```python
from build123d import *

# Parameters (mm, degrees)
ESQUISSE1_R             = 35
ESQUISSE1_R_2           = 7
BOSS_EXTRU_1_DEPTH      = 20
ESQUISSE2_R             = 14
ENL_V_MAT_EXTRU_1_DEPTH = 5
ESQUISSE3_R             = 4
ENL_V_MAT_EXTRU_3_DEPTH = 5
ESQUISSE8_R             = 14
ENL_V_MAT_EXTRU_4_DEPTH = 25
BOSS_EXTRU_2_DEPTH      = 6
BOSS_EXTRU_2_DEPTH_BACK = 9
ESQUISSE9_R             = 4
ESQUISSE10_R            = 14
ESQUISSE10_R_2          = 10.5
BOSS_EXTRU_3_DEPTH      = 20


with BuildPart() as part:
    # Esquisse1 → Boss.-Extru.1 (new body)
    with BuildSketch(Plane.XY):
        Circle(ESQUISSE1_R)
        Circle(ESQUISSE1_R_2, mode=Mode.SUBTRACT)
    extrude(amount=BOSS_EXTRU_1_DEPTH)

    # Esquisse2 → Enlèv. mat.-Extru.1 (cut)
    with BuildSketch(Plane(origin=(0, 0, 0), x_dir=(-1, 0, 0), z_dir=(0, 0, -1))):
        Circle(ESQUISSE2_R)
    extrude(amount=-ENL_V_MAT_EXTRU_1_DEPTH, mode=Mode.SUBTRACT)

    # Esquisse3 → Enlèv. mat.-Extru.3 (cut)
    with BuildSketch(Plane(origin=(0, 0, 0), x_dir=(-1, 0, 0), z_dir=(0, 0, -1))):
        with Locations((-13.588993608, 22.602101614)):
            Circle(ESQUISSE3_R)
        with Locations((13.588993608, 22.602101614)):
            Circle(ESQUISSE3_R)
        with Locations((26.369096609, 0.431843358)):
            Circle(ESQUISSE3_R)
        with Locations((12.841601354, -23.034952123)):
            Circle(ESQUISSE3_R)
        with Locations((-12.82933858, -23.041784138)):
            Circle(ESQUISSE3_R)
        with Locations((-26.369096609, 0.431843358)):
            Circle(ESQUISSE3_R)
    extrude(amount=-ENL_V_MAT_EXTRU_3_DEPTH, mode=Mode.SUBTRACT)

    # Esquisse8 → Enlèv. mat.-Extru.4 (cut)
    with BuildSketch(Plane(origin=(0, 0, 0), x_dir=(-1, 0, 0), z_dir=(0, 0, -1))):
        Circle(ESQUISSE8_R)
    extrude(amount=-ENL_V_MAT_EXTRU_4_DEPTH, mode=Mode.SUBTRACT)

    # Esquisse9 → Boss.-Extru.2 (add, two sides: drawn at the far end of the back side and taken through both)
    with BuildSketch(Plane(origin=(0, 0, 0), x_dir=(-1, 0, 0), z_dir=(0, 0, -1)).offset(-BOSS_EXTRU_2_DEPTH_BACK)):
        with Locations((-13.588993608, 22.602101614)):
            Circle(ESQUISSE9_R)
        with Locations((13.588993608, 22.602101614)):
            Circle(ESQUISSE9_R)
        with Locations((26.369096609, 0.431843358)):
            Circle(ESQUISSE9_R)
        with Locations((12.841601354, -23.034952123)):
            Circle(ESQUISSE9_R)
        with Locations((-12.82933858, -23.041784138)):
            Circle(ESQUISSE9_R)
        with Locations((-26.369096609, 0.431843358)):
            Circle(ESQUISSE9_R)
    extrude(amount=BOSS_EXTRU_2_DEPTH + BOSS_EXTRU_2_DEPTH_BACK)

    # Esquisse10 → Boss.-Extru.3 (add)
    with BuildSketch(Plane(origin=(0, 0, 0), x_dir=(-1, 0, 0), z_dir=(0, 0, -1))):
        Circle(ESQUISSE10_R)
        Circle(ESQUISSE10_R_2, mode=Mode.SUBTRACT)
    extrude(amount=-BOSS_EXTRU_3_DEPTH)


solid = part.part
```
Model file for the job. Use its own axes, mm. A direction names the side the tool comes from. Give positions to 0.01 mm unless a question says otherwise; leave off trailing zeros. Order: outer loops, then holes, each group sorted by start corner. A loop starts at its lowest first (then second) coordinate and runs counter-clockwise, first axis right, second up.
1) Saw through at D-D, the plane x = 14.5. Write the cut outline in (y, z), then the cut area to 3 significant figures.
2) Saw through at B-B, the plane z = -1.75. Write the cut outline in (x, y), then the cut area to 3 significant figures.
3) Mould opens along X. For faces 3 (the cylindrical face through (22.674, -1.1, -2.958)), 4 (the cylindrical face through (9.014, -21.84, -2.958)), 5 (the flat face through (14, 23, -6)), 6 (the cylindrical face through (-28, -21, 10)) say: +X half, -X half, draft (parallel to the pull), parting line (faces both ways), or undercut.
4) Saw through at C-C, the plane y = -2. Write the cut outline in (x, z).
5) Pin check, flat tips, straight feed: pin 1 (6 mm diameter, centred on x = -4.5, z = 9.5, fed in from -Y); pin 2 (1.5 mm diameter, centred on y = 21, z = 14, fed in from -X); pin 3 (2 mm diameter, centred on x = -4.5, z = 0, fed in from -Y); pin 4 (17 mm diameter, centred on x = 0, y = 0, fed in from -Z). Stop position of each tip, or through.
6) Wall check: probe 1 along Y at (x, z) = (0, 5); probe 2 along Z at (x, y) = (7, 22.5); probe 3 along Y at (x, z) = (5.5, 6.75). Give the ranges that are in metal, low to high.
7) 3-axis set-ups, long thin cutter, end or side, ignore diameter. For faces 1 (the flat face through (-26, 0, -6)), 2 (the flat face through (8.3, -7.3, 0)): which of +Z, -Z, +X, -X, +Y, -Y reach the whole face in a straight line?
8) Saw through at A-A, the plane x = 0. Write the cut outline in (y, z).
Computed:
1. outline: (-31.86, 0) - (-26.68, 0) - (-26.68, -6) - (-19.41, -6) - (-19.41, 0) - (18.71, 0) - (18.71, -6) - (26.5, -6) - (26.5, 0) - (31.86, 0) - (31.86, 20) - (-31.86, 20) - close
1. area: 1,360 mm2
2. outline: circle Ø8 at (-26.37, 0.43); circle Ø8 at (-13.59, 22.6); circle Ø8 at (-12.84, -23.03); circle Ø8 at (12.83, -23.04); circle Ø8 at (13.59, 22.6); circle Ø8 at (26.37, 0.43)
2. area: 302 mm2
3. face 3: undercut
3. face 4: undercut
3. face 5: draft
3. face 6: parting line
4. outline: (-34.94, 0) - (-29.54, 0) - (-29.54, -6) - (-23.19, -6) - (-23.19, 0) - (-10.31, 0) - (-10.31, 20) - (-34.94, 20) - close; (10.31, 0) - (23.19, 0) - (23.19, -6) - (29.54, -6) - (29.54, 0) - (34.94, 0) - (34.94, 20) - (10.31, 20) - close
5. pin 1: stops at y = -34.97
5. pin 2: stops at x = -28.55
5. pin 3: stops at y = -34.82
5. pin 4: passes through
6. probe 1: y = -35 to -10.5, 10.5 to 35
6. probe 2: z = 0 to 20
6. probe 3: y = -34.57 to -8.94, 8.94 to 34.57
7. face 1: -Z, +X, -X, +Y, -Y
7. face 2: -Z
8. outline: (-35, 0) - (-10.5, 0) - (-10.5, 20) - (-35, 20) - close; (10.5, 0) - (35, 0) - (35, 20) - (10.5, 20) - close
